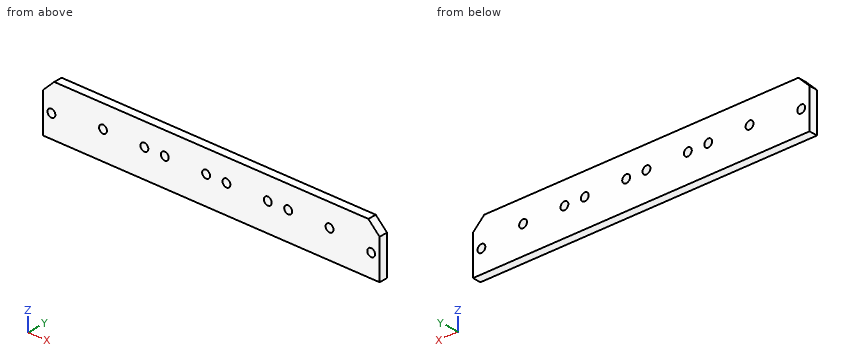
from build123d import *

# Parameters (mm, degrees)
SKETCH_1_W          = 120
SKETCH_1_H          = 35
EXTRUDE_1_DEPTH     = 3
SKETCH_2_W          = 30
SKETCH_2_H          = 17
CUT_EXTRUDE_1_DEPTH = 63.571958576
SKETCH_3_R          = 1.4
CUT_EXTRUDE_2_DEPTH = 63.571958576
SKETCH_4_R          = 1.4
CUT_EXTRUDE_3_DEPTH = 63.571958576
SKETCH_5_W          = 10
SKETCH_5_H          = 5
CUT_EXTRUDE_4_DEPTH = 63.571958576
CHAMFER_1_SIZE      = 4
CHAMFER_1_SIZE2     = 8.578027682
CHAMFER_2_SIZE      = 4
CHAMFER_2_SIZE2     = 8.578027682
FILLET_1_R          = 5
CHAMFER_3_SIZE      = 4
SKETCH_6_W          = 120
SKETCH_6_H          = 17
CUT_EXTRUDE_5_DEPTH = 63.571958576


with BuildPart() as part:
    # 草图1 → 凸台-拉伸1 (new body)
    with BuildSketch(Plane(origin=(0, 0, 0), x_dir=(1, 0, 0), z_dir=(0, 1, 0))):
        Rectangle(SKETCH_1_W, SKETCH_1_H)
    extrude(amount=EXTRUDE_1_DEPTH)

    # 草图2 → 切除-拉伸1 (cut, through all)
    with BuildSketch(Plane(origin=(0, 3, 0), x_dir=(1, 0, 0), z_dir=(0, 1, 0))):
        with Locations((0, 9)):
            Rectangle(SKETCH_2_W, SKETCH_2_H)
    extrude(amount=-CUT_EXTRUDE_1_DEPTH, mode=Mode.SUBTRACT)

    # 草图3 → 切除-拉伸2 (cut, through all)
    with BuildSketch(Plane(origin=(0, 3, 0), x_dir=(1, 0, 0), z_dir=(0, 1, 0))):
        with Locations(Location((-57, 12.5, 0), (0, 0, 270))):
            Circle(SKETCH_3_R)
        with Locations(Location((-57, -7.5, 0), (0, 0, 270))):
            Circle(SKETCH_3_R)
        with Locations(Location((57, -7.5, 0), (0, 0, 90))):
            Circle(SKETCH_3_R)
        with Locations(Location((57, 12.5, 0), (0, 0, 90))):
            Circle(SKETCH_3_R)
    extrude(amount=-CUT_EXTRUDE_2_DEPTH, mode=Mode.SUBTRACT)

    # 草图4 → 切除-拉伸3 (cut, through all)
    with BuildSketch(Plane(origin=(0, 3, 0), x_dir=(1, 0, 0), z_dir=(0, 1, 0))):
        with Locations(Location((5.4, -9.5, 0), (0, 0, 270))):
            Circle(SKETCH_4_R)
        with Locations(Location((20.15, -9.5, 0), (0, 0, 270))):
            Circle(SKETCH_4_R)
        with Locations(Location((27.4, -9.5, 0), (0, 0, 270))):
            Circle(SKETCH_4_R)
        with Locations(Location((42.15, -9.5, 0), (0, 0, 270))):
            Circle(SKETCH_4_R)
        with Locations(Location((-1.85, -9.5, 0), (0, 0, 270))):
            Circle(SKETCH_4_R)
        with Locations(Location((-16.6, -9.5, 0), (0, 0, 270))):
            Circle(SKETCH_4_R)
        with Locations(Location((-23.85, -9.5, 0), (0, 0, 270))):
            Circle(SKETCH_4_R)
        with Locations(Location((-38.6, -9.5, 0), (0, 0, 270))):
            Circle(SKETCH_4_R)
    extrude(amount=-CUT_EXTRUDE_3_DEPTH, mode=Mode.SUBTRACT)

    # 草图5 → 切除-拉伸4 (cut, through all)
    with BuildSketch(Plane(origin=(0, 3, 0), x_dir=(1, 0, 0), z_dir=(0, 1, 0))):
        with Locations((-30, 7.5)):
            Rectangle(SKETCH_5_W, SKETCH_5_H)
        with Locations((30, 7.5)):
            Rectangle(SKETCH_5_W, SKETCH_5_H)
    extrude(amount=-CUT_EXTRUDE_4_DEPTH, mode=Mode.SUBTRACT)

    # 倒角1
    chamfer_1_edges = [part.edges().sort_by_distance(p)[0] for p in [
        (-15, 1.5, -17.5),
    ]]
    chamfer_1_side = [part.faces().sort_by_distance(p)[0] for p in [
        (-37.5, 1.5, -17.5),
    ]]
    chamfer(chamfer_1_edges, length=CHAMFER_1_SIZE, length2=CHAMFER_1_SIZE2, reference=chamfer_1_side[0])

    # 倒角2
    chamfer_2_edges = [part.edges().sort_by_distance(p)[0] for p in [
        (15, 1.5, -17.5),
    ]]
    chamfer_2_side = [part.faces().sort_by_distance(p)[0] for p in [
        (37.5, 1.5, -17.5),
    ]]
    chamfer(chamfer_2_edges, length=CHAMFER_2_SIZE, length2=CHAMFER_2_SIZE2, reference=chamfer_2_side[0])

    # 圆角1
    fillet_1_edges = [part.edges().sort_by_distance(p)[0] for p in [
        (-15, 1.5, -0.5),
        (15, 1.5, -0.5),
    ]]
    fillet(fillet_1_edges, radius=FILLET_1_R)

    # 倒角3
    chamfer_3_edges = [part.edges().sort_by_distance(p)[0] for p in [
        (60, 1.5, 17.5),
        (-60, 1.5, 17.5),
    ]]
    chamfer(chamfer_3_edges, length=CHAMFER_3_SIZE)

    # 草图6 → 切除-拉伸5 (cut, through all)
    with BuildSketch(Plane(origin=(0, 3, 0), x_dir=(1, 0, 0), z_dir=(0, 1, 0))):
        with Locations((0, 9)):
            Rectangle(SKETCH_6_W, SKETCH_6_H)
    extrude(amount=-CUT_EXTRUDE_5_DEPTH, mode=Mode.SUBTRACT)


solid = part.part
Source: CAD feature listing. Evaluate the final solid. Frame: model axes, mm. Give positions to 0.01 mm unless a question says otherwise; leave off trailing zeros. Write each loop counter-clockwise with the first axis right and the second up, starting at its lowest first coordinate (ties: lowest second). Pieces come first, ordered by that corner, then holes. Notation, with made-up numbers: M 70,30.25 L 84,30.25 A25 ccw 84,58.25 Z; hole C 54,-23 d3. An arc over 180 degrees is marked long. Return JSON: item names as keys, results as strings. Group by question number.
1) Cut plane B-B, the plane y = 0.8. Give the number of separate pieces and of enclosed holes in the cut face, then the cut area to 3 significant figures.
2) Ray query, L1, parallel to X at y = 2.45, z = 7.5; L2, parallel to Z at x = 27.5, y = 0.75; L3, parallel to X at y = 1.8, z = 6.75. Return the intervals inside material, ascending.
3) Cut plane C-C, the plane x = 42.15. Output: boundary loops of the cut face in (y, z).
4) Cut plane A-A, the plane x = 57. Output: boundary loops of the cut face in (y, z), then the cut area to 3 significant figures.
Data:
{
 "1": {"separate pieces": "1", "enclosed holes": "10", "area": "2,080 mm²"},
 "2": {"L1": "x = -60 to -58.4, -55.6 to 55.6, 58.4 to 60", "L2": "z = -0.5 to 8.1, 10.9 to 17.5", "L3": "x = -60 to -58.18, -55.82 to 55.82, 58.18 to 60"},
 "3": {"outline": "M 0,-0.5 L 3,-0.5 L 3,8.1 L 0,8.1 Z; M 0,10.9 L 3,10.9 L 3,17.5 L 0,17.5 Z"},
 "4": {"outline": "M 0,-0.5 L 3,-0.5 L 3,6.1 L 0,6.1 Z; M 0,8.9 L 3,8.9 L 3,16.5 L 0,16.5 Z", "area": "42.6 mm²"}
}
